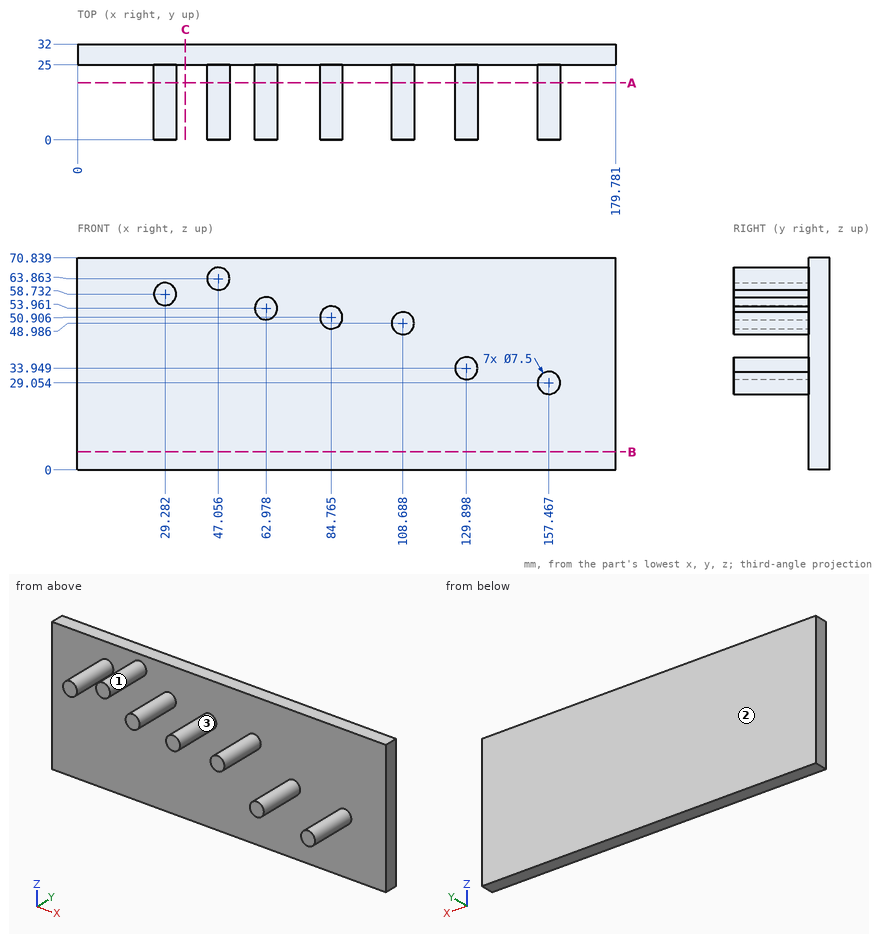
Check sheet for the drawn part. Datum: minimum x, y, z corner. Units: mm. Round coordinates to 2 decimals unless told otherwise and drop trailing zeros. Order: outer loops, then holes, each group sorted by start corner. A loop starts at its lowest first (then second) coordinate and runs counter-clockwise, first axis right, second up.
(1) Scan lines: probe 1 along Y at (x, z) = (128, 54); probe 2 along X at (y, z) = (4, 34); probe 3 along Z at (x, y) = (84.5, 10) (1 decimal). Record each from-to range of solid material in increasing order.
(2) Cross-section at B-B, the plane z = 6. Enter the section's corners in (x, y), and give its area (3 significant figures).
(3) Cross-section at C-C, the plane x = 36. Enter the section's corners in (y, z), and give its area (3 significant figures).
(4) Go/stop test with flat-tipped pins: P1, Ø2, axis at x = 86.5, z = 28, coming from the -Y side; P2, Ø1.5, axis at x = 159, y = 18.5, coming from the -Z side; P3, Ø1.5, axis at y = 23.5, z = 26, coming from the +X side (1 decimal); P4, Ø8, axis at x = 76.5, y = 10, coming from the -Z side. Record where each tip stops, or that it passes through.
(5) Cross-section at A-A, the plane y = 19. State how many separate pieces and enclosed holes the cut face has, and give its area (3 significant figures).
(6) Draft check along X on the marked faces 1, 2 and 3. Enter one of: pulls with the +X half, pulls with the -X half, needs draft (parallel to the pull), parting line crosses it, or undercut.
Check sheet entries:
1. probe 1: y = 25 to 32
1. probe 2: x = 126.15 to 133.65
1. probe 3: z = 47.2 to 54.6
2. outline: (0, 25) - (179.78, 25) - (179.78, 32) - (0, 32) - close
2. area: 1,260 mm2
3. outline: (25, 0) - (32, 0) - (32, 70.84) - (25, 70.84) - close
3. area: 496 mm2
4. P1: stops at y = 25
4. P2: stops at z = 25.39
4. P3: stops at x = 160.4
4. P4: passes through
5. separate pieces: 7
5. enclosed holes: 0
5. area: 309 mm2
6. face 1: undercut
6. face 2: needs draft
6. face 3: undercut
